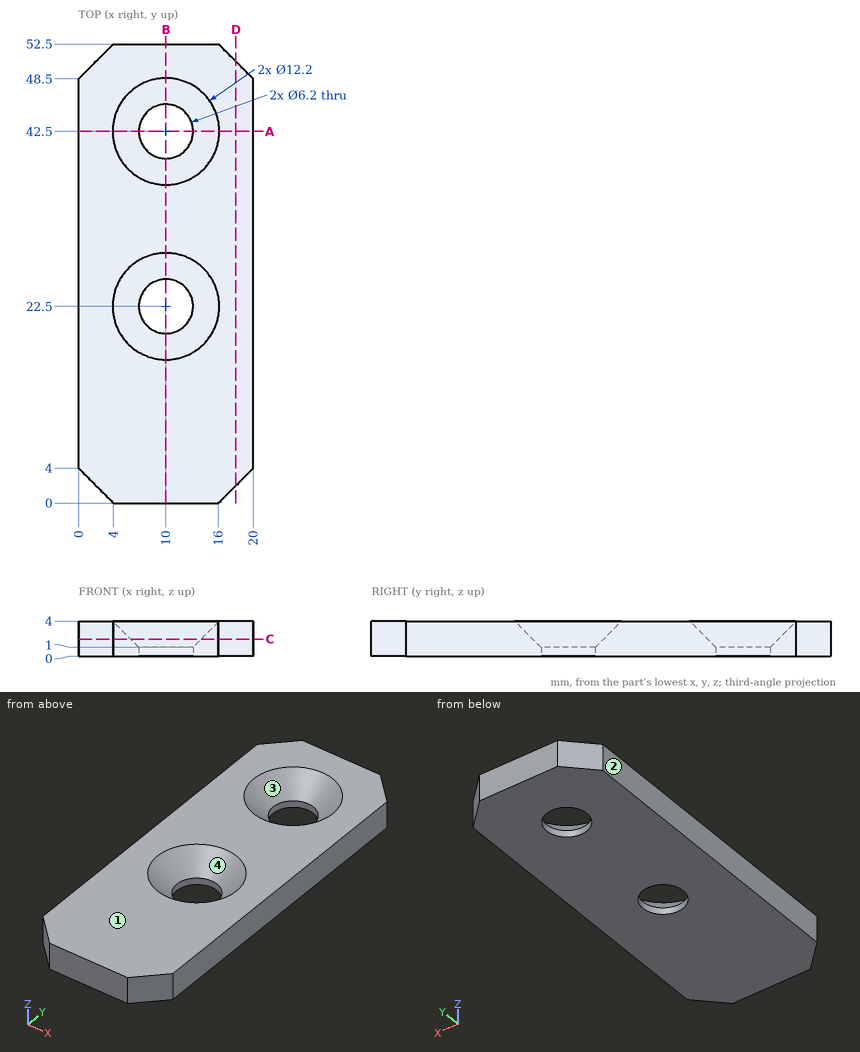
Geometry check sheet. Reference: drawing and pictorial views, mm from the part's lowest x, y, z. Give positions to 0.01 mm unless a question says otherwise; leave off trailing zeros. Write each loop counter-clockwise with the first axis right and the second up, starting at its lowest first coordinate (ties: lowest second). Pieces come first, ordered by that corner, then holes. Notation, with made-up numbers: M 30,25.5 L 37,25.5 A21 cw 37,62.5 Z; hole C 89.5,4.25 d10. An arc over 180 degrees is marked long. Use CSV: the item, a comma, the result in double quotes.
1) Cross-section at B-B (x = 10). Enter the section's corners in (y, z), plus the area to 3 significant figures.
Final values:
outline,"M 0,0 L 19.4,0 L 19.4,1 L 16.4,4 L 0,4 Z; M 25.6,0 L 39.4,0 L 39.4,1 L 36.4,4 L 28.6,4 L 25.6,1 Z; M 45.6,0 L 52.5,0 L 52.5,4 L 48.6,4 L 45.6,1 Z"
area,"142 mm²"
2) Cross-section at D-D (x = 18). Enter the section's corners in (y, z), plus the area to 3 significant figures.
Final values:
outline,"M 2,0 L 50.5,0 L 50.5,4 L 2,4 Z"
area,"194 mm²"
3) Release check for a two-part mould opening along X. For the marked faces 1, 2, 3 and 4 record: released by +X, released by -X, zero draft, split by the parting line, or undercut.
Final values:
face 1,"zero draft"
face 2,"released by -X"
face 3,"undercut"
face 4,"undercut"
4) Material ranges on line 1 along Y through (x, z) = (10, 0.5); line 2 along X through (y, z) = (43, 0.4); line 3 along X through (y, z) = (20.5, 0.3), recorded low to high.
Final values:
line 1,"0 to 19.4, 25.6 to 39.4, 45.6 to 52.5"
line 2,"0 to 6.94, 13.06 to 20"
line 3,"0 to 7.63, 12.37 to 20"
5) Cross-section at C-C (z = 1.95). Enter the section's corners in (x, y).
Final values:
outline,"M 0,4 L 4,0 L 16,0 L 20,4 L 20,48.5 L 16,52.5 L 4,52.5 L 0,48.5 Z; hole C 10,22.5 d8.1; hole C 10,42.5 d8.1"
6) Cross-section at A-A (y = 42.5). Enter the section's corners in (x, z), plus the area to 3 significant figures.
Final values:
outline,"M 0,0 L 6.9,0 L 6.9,1 L 3.9,4 L 0,4 Z; M 13.1,0 L 20,0 L 20,4 L 16.1,4 L 13.1,1 Z"
area,"46.2 mm²"
